Here's how the part is built. I have some questions about the finished solid (model axes, mm). A direction names the side the tool comes from. Coordinates: 2 decimals unless noted, no trailing zeros. Order: outer loops, then holes, each group sorted by start corner. A loop starts at its lowest first (then second) coordinate and runs counter-clockwise, first axis right, second up. Notation, with made-up numbers: (12, 54.5) - (16, 54.5) arc R4 cw to (16, 60.5) - close; hole circle Ø8 at (58.5, 20.25). An arc over 180 degrees is marked (long way). Answer in a Markdown table with one row per item. Add a question column.
Item 1: I want a section at C-C (y = 22.25). Please give me the cut outline in (x, z), plus the area to 3 significant figures.
Item 2: Will these pins go through, and if not, where does the flat tip stop? pin 1 Ø2 at (x, z) = (9.5, 3.5) entering from +Y; pin 2 Ø2.5 at (x, z) = (13, 8) entering from +Y; pin 3 Ø5 at (y, z) = (22.5, 2.5) entering from -X.
Item 3: On a 3-axis mill with a long thin cutter (end or side, diameter ignored), from which of +Z, -Z, +X, -X, +Y, -Y can I reach the whole of each face in a straight line? I mean faces 1 (the cylindrical face through (5.363, 27.454, 4.715)), 2 (the flat face through (-11.35, 19, 6)), 3 (the flat face through (10, 20.4, 2)), 4 (the flat face through (10, 20.4, 11)). Say none if no direction works.
Item 4: I want a section at B-B (x = -7). Please give me the cut outline in (y, z).
Item 5: I want a section at A-A (y = 11.5). Please give me the cut outline in (x, z), plus the area to 3 significant figures.
Item 6: If I drill on line 1 along X through (y, z) = (13.75, 11); line 2 along Y through (x, z) = (-6, 7); line 3 along Y through (x, z) = (7.5, 1), over which ranges is the centre line in solid material (lowest first)? Write a range as from..to.
```python
from build123d import *

# Parameters (mm, degrees)
F3_DEPTH  = 12.7
F4_R      = 0.5
F6_R      = 6.35
F7_DEPTH  = 5.6
F8_R      = 0.5
F9_R      = 1.6747204535
F10_DEPTH = 2.95


with BuildPart() as f3:
    # F2 (on Top) → F3 (new body)
    with BuildSketch(Plane.XY):
        Polygon((11.35, 20.4), (-11.35, 20.4), (-11.35, 17.55), (-15.92, 17.55), (-15.92, 15.4), (-11.35, 15.4), (-11.35, 0), (11.35, 0), (11.35, 15.4), (15.92, 15.4), (15.92, 17.55), (11.35, 17.55), align=None)
    extrude(amount=F3_DEPTH)

    # F4
    f4_edges = [f3.edges().sort_by_distance(p)[0] for p in [
        (11.35, 7.7, 12.7),
        (11.35, 18.975, 12.7),
        (11.35, 18.975, 0),
        (11.35, 7.7, 0),
        (-11.35, 18.975, 12.7),
        (-11.35, 7.7, 12.7),
        (-11.35, 18.975, 0),
        (-11.35, 7.7, 0),
    ]]
    fillet(f4_edges, radius=F4_R)

    # F6 (on offset) → F7 (join)
    with BuildSketch(Plane(origin=(0, 20.4, 0), x_dir=(-1, 0, 0), z_dir=(0, 1, 0))):
        with Locations((-5, 6.35)):
            Circle(F6_R)
    extrude(amount=F7_DEPTH)

    # F8
    f8_edges = [f3.edges().sort_by_distance(p)[0] for p in [
        (11.35, 26, 6.35),
    ]]
    fillet(f8_edges, radius=F8_R)

    # F9 (on face) → F10 (join)
    with BuildSketch(Plane(origin=(0, 26, 0), x_dir=(-1, 0, 0), z_dir=(0, 1, 0))):
        with Locations((-5, 6.35)):
            Circle(F9_R)
    extrude(amount=F10_DEPTH)


solid = f3.part
```
Values follow:
| question | item | result |
|---|---|---|
| 1 | outline | circle Ø12.7 at (5, 6.35) |
| 1 | area | 127 mm^2 |
| 2 | pin 1 | stops at y = 26 |
| 2 | pin 2 | stops at y = 17.55 |
| 2 | pin 3 | stops at x = -11.35 |
| 3 | face 1 | +Y |
| 3 | face 2 | +Z, -Z, -X, +Y |
| 3 | face 3 | -Z, +X, +Y |
| 3 | face 4 | +Z, +X, +Y |
| 4 | outline | (0, 0) - (20.4, 0) - (20.4, 12.7) - (0, 12.7) - close |
| 5 | outline | (-11.35, 0.5) arc R0.5 ccw to (-10.85, 0) - (10.85, 0) arc R0.5 ccw to (11.35, 0.5) - (11.35, 12.2) arc R0.5 ccw to (10.85, 12.7) - (-10.85, 12.7) arc R0.5 ccw to (-11.35, 12.2) - close |
| 5 | area | 288 mm^2 |
| 6 | line 1 | x = -11.35..11.35 |
| 6 | line 2 | y = 0..20.4 |
| 6 | line 3 | y = 0..26 |
